```python
from build123d import *

# Parameters (mm, degrees)
EXTRUDE_1_DEPTH             = 9.2
SKETCH_2_W                  = 162.4
SKETCH_2_H                  = 18.4
EXTRUDE_2_DEPTH             = 40
HOLE_WIZARD_M82_D           = 8.4
HOLE_WIZARD_M82_CBORE_D     = 15
HOLE_WIZARD_M82_CBORE_DEPTH = 8
HOLE_WIZARD_6_0_6_2_D       = 6


with BuildPart() as part:
    # Эскиз1 → Бобышка-Вытянуть1 (new, symmetric)
    with BuildSketch(Plane.XY):
        Polygon((-69.2, -12), (-30.426406871, -12), (-6, -36.426406871), (-6, -47), (6, -47), (6, -36.426406871), (30.426406871, -12), (69.2, -12), (69.2, -60), (-69.2, -60), align=None)
    extrude(amount=EXTRUDE_1_DEPTH, both=True)

    # Эскиз2 → Бобышка-Вытянуть2 (add)
    with BuildSketch(Plane.XZ.offset(60)):
        Rectangle(SKETCH_2_W, SKETCH_2_H)
    extrude(amount=EXTRUDE_2_DEPTH)

    # Цековка для винта с внутренним шестигранником M82 (through all)
    with Locations(Plane(origin=(0, -12, 0), x_dir=(-1, 0, 0), z_dir=(0, 1, 0))):
        with Locations((-60, 0.343824936), (60, -0.343824936)):
            CounterBoreHole(HOLE_WIZARD_M82_D / 2, HOLE_WIZARD_M82_CBORE_D / 2, HOLE_WIZARD_M82_CBORE_DEPTH)

    # Диаметр отверстия Ø6.0 (6)2 (through all)
    with Locations(Plane(origin=(0, -60, 0), x_dir=(-1, 0, 0), z_dir=(0, 1, 0))):
        with Locations((-75.2, 0), (75.2, 0)):
            Hole(HOLE_WIZARD_6_0_6_2_D / 2)


solid = part.part
```
The listing builds one solid part. Answer for the finished solid, in the listing's coordinates (mm). A direction names the side the tool comes from. Coordinates: 2 decimals unless noted, no trailing zeros. Loops run counter-clockwise (first coordinate to the right, second up) from the corner with the lowest first, then second, coordinate; pieces in that order, holes last. Notation, with made-up numbers: (41, 20) - (98, 20) arc R7 cw to (98, 32) - close; hole circle Ø6 at (-8, 14.25). An arc over 180 degrees is marked (long way). Write item = value, one per line.
1) Find the intervals of material crossed by line 1 along Z through (x, y) = (-75.2, -76); line 2 along Z through (x, y) = (-60, -16); line 3 along X through (y, z) = (-75.5, -0.5), in increasing order.
Responses:
line_1 = -9.2 to -3, 3 to 9.2
line_2 = -9.2 to -7.84, 7.16 to 9.2
line_3 = -81.2 to -78.16, -72.24 to -64.2, -55.8 to 55.89, 64.11 to 72.24, 78.16 to 81.2
2) Section C-C (y = -85) is taken. Determine the outline of the cut face in (x, z), plus the area to 3 significant figures.
Responses:
outline = (-81.2, -9.2) - (81.2, -9.2) - (81.2, 9.2) - (-81.2, 9.2) - close; hole circle Ø6 at (-75.2, 0); hole circle Ø8.4 at (-60, -0.34); hole circle Ø8.4 at (60, 0.34); hole circle Ø6 at (75.2, 0)
area = 2,820 mm^2
3) Section A-A (y = -44.5) is taken. Determine the outline of the cut face in (x, z).
Responses:
outline = (-69.2, -9.2) - (-6, -9.2) - (-6, 9.2) - (-69.2, 9.2) - close; (6, -9.2) - (69.2, -9.2) - (69.2, 9.2) - (6, 9.2) - close; hole circle Ø8.4 at (-60, -0.34); hole circle Ø8.4 at (60, 0.34)
4) Section B-B (x = 60) is taken. Determine the outline of the cut face in (y, z).
Responses:
outline = (-100, -9.2) - (-12, -9.2) - (-12, -7.16) - (-20, -7.16) - (-20, -3.86) - (-100, -3.86) - close; (-100, 4.54) - (-20, 4.54) - (-20, 7.84) - (-12, 7.84) - (-12, 9.2) - (-100, 9.2) - close
5) Section D-D (y = -23.5) is taken. Determine the outline of the cut face in (x, z).
Responses:
outline = (-69.2, -9.2) - (-18.93, -9.2) - (-18.93, 9.2) - (-69.2, 9.2) - close; (18.93, -9.2) - (69.2, -9.2) - (69.2, 9.2) - (18.93, 9.2) - close; hole circle Ø8.4 at (-60, -0.34); hole circle Ø8.4 at (60, 0.34)
6) Determine the mould class of faces 6 (the face through (45, -12, 0)), 7 (the face through (-81.2, -80, 0)), 8 (the face through (57, -20, -3)) for opening direction X: pulls with the +X half, pulls with the -X half, needs draft (parallel to the pull), parting line crosses it, or undercut.
Responses:
face_6 = needs draft
face_7 = pulls with the -X half
face_8 = undercut
7) Which of the six approach directions +Z, -Z, +X, -X, +Y, -Y give full straight-line access (tool end or side, diameter ignored) to faces 1 (the face through (-1, -65, 9.2)), 2 (the face through (-69.2, -36, 0)), 3 (the face through (-52.507, -15.944, -0.014)), 4 (the face through (6, -42, 0)), 5 (the face through (69.2, -36, 0))?
Responses:
face_1 = +Z, +X, -X, +Y, -Y
face_2 = +Z, -Z, -X, +Y
face_3 = +Y
face_4 = +Z, -Z, +Y
face_5 = +Z, -Z, +X, +Y
8) Each of these flat-tipped pins is pushed along its axis until it touches: P1, Ø3, axis at x = -22, z = 4, coming from the +Y side; P2, Ø9, axis at y = -27.5, z = 1, coming from the +X side; P3, Ø7.5, axis at x = 59.5, z = -0.5, coming from the +Y side. Where does it stop, or does it pass through?
Responses:
P1 = -18.93
P2 = 69.2
P3 = -20
